Design review of the part built by this model. Coordinates are the model's own, in mm. Face numbers are marked on the shaded views. A direction names the side the tool comes from. Give positions to 0.01 mm unless a question says otherwise; leave off trailing zeros. Write each loop counter-clockwise with the first axis right and the second up, starting at its lowest first coordinate (ties: lowest second). Pieces come first, ordered by that corner, then holes. Notation, with made-up numbers: (-22.75, 59.25) -> (31.25, 59.25) arc R18 cw to (31.25, 80.25) -> close; hole circle Ø3 at (-11.75, -20.5). An arc over 180 degrees is marked (long way). Write each question's results on one line, items separated by ' | '. Start each with the question number.
(1) For the marked faces 4 and 5, list the 3-axis set-ups (+Z, -Z, +X, -X, +Y, -Y) from which the entire face can be reached by the end or side of a thin tool; tool diameter is ignored.
(2) To check wall thickness, follow probe 1 along X at (y, z) = (3, 18.25); probe 2 along Y at (x, z) = (13, 17); probe 3 along Z at (x, y) = (-26.5, -6). State the ranges of each line that lie inside material, in increasing order.
(3) Take a section at B-B (x = 3). Count the separate pieces of the cut face and the enclosed holes in it, plus the area to 3 significant figures.
(4) Take a section at C-C (y = 8.5). State the section outline as (x, z) points, plus the area to 3 significant figures.
(5) Take a section at A-A (z = 17.75). State the section outline as (x, y) points, plus the area to 3 significant figures.
(6) Mouldability with a two-part tool opening along Y and no side actions: class the marked faces 1, 2 and 3 as released by +Y, released by -Y, zero draft, split by the parting line, or undercut.
(7) Clearance check with flat-ended pins moving along their axes: pin 1 (6 mm diameter, centred on y = 3.5, z = 11.5, fed in from -X); pin 2 (1.2 mm diameter, centred on x = 30.5, y = -8.5, fed in from -Z). State where each tip first meets the part, or that it passes through.
from build123d import *

# Parameters (mm, degrees)
SKETCH1_W           = 61.7
SKETCH1_H           = 31.7
SKETCH1_W_2         = 58.7
SKETCH1_H_2         = 28.7
BOSS_EXTRUDE1_DEPTH = 19
SKETCH2_W           = 61.7
SKETCH2_H           = 31.7
BOSS_EXTRUDE2_DEPTH = 1
BOSS_EXTRUDE3_DEPTH = 5
CUT_EXTRUDE4_DEPTH  = 2
CUT_EXTRUDE2_DEPTH  = 32.7
CUT_EXTRUDE3_DEPTH  = 62.7
SKETCH9_W           = 7
SKETCH9_H           = 8.75
CUT_EXTRUDE5_DEPTH  = 62.7


with BuildPart() as part:
    # Sketch1 → Boss-Extrude1 (new body)
    with BuildSketch(Plane.XY):
        Rectangle(SKETCH1_W, SKETCH1_H)
        Rectangle(SKETCH1_W_2, SKETCH1_H_2, mode=Mode.SUBTRACT)
    extrude(amount=BOSS_EXTRUDE1_DEPTH)

    # Sketch2 → Boss-Extrude2 (add)
    with BuildSketch(Plane.XY.offset(19)):
        Rectangle(SKETCH2_W, SKETCH2_H)
    extrude(amount=BOSS_EXTRUDE2_DEPTH)

    # Sketch3 → Boss-Extrude3 (add)
    with BuildSketch(Plane(origin=(0, 0, 0), x_dir=(-1, 0, 0), z_dir=(0, 0, -1))):
        Polygon((-30.85, -15.85), (30.85, -15.85), (30.85, 15.85), (9, 15.85), (9, 14.35), (29.35, 14.35), (29.35, -14.35), (-29.35, -14.35), (-29.35, 14.35), (-9, 14.35), (-9, 15.85), (-30.85, 15.85), align=None)
    extrude(amount=BOSS_EXTRUDE3_DEPTH)

    # Sketch8 → Cut-Extrude4 (cut, through all)
    with BuildSketch(Plane(origin=(0, 0, 19), x_dir=(-1, 0, 0), z_dir=(0, 0, -1))):
        with BuildLine():
            Line((12, 6.5), (22, 6.5))
            ThreePointArc((22, 6.5), (24, 8.5), (22, 10.5))
            Line((22, 10.5), (12, 10.5))
            ThreePointArc((12, 10.5), (10, 8.5), (12, 6.5))
        make_face()
        with BuildLine():
            Line((12, -2), (22, -2))
            ThreePointArc((22, -2), (24, 0), (22, 2))
            Line((22, 2), (12, 2))
            ThreePointArc((12, 2), (10, 0), (12, -2))
        make_face()
        with BuildLine():
            Line((12, -10.5), (22, -10.5))
            ThreePointArc((22, -10.5), (24, -8.5), (22, -6.5))
            Line((22, -6.5), (12, -6.5))
            ThreePointArc((12, -6.5), (10, -8.5), (12, -10.5))
        make_face()
        with BuildLine():
            Line((-5, -10.5), (5, -10.5))
            ThreePointArc((5, -10.5), (7, -8.5), (5, -6.5))
            Line((5, -6.5), (-5, -6.5))
            ThreePointArc((-5, -6.5), (-7, -8.5), (-5, -10.5))
        make_face()
        with BuildLine():
            Line((-22, -10.5), (-12, -10.5))
            ThreePointArc((-12, -10.5), (-10, -8.5), (-12, -6.5))
            Line((-12, -6.5), (-22, -6.5))
            ThreePointArc((-22, -6.5), (-24, -8.5), (-22, -10.5))
        make_face()
        with BuildLine():
            Line((-22, -2), (-12, -2))
            ThreePointArc((-12, -2), (-10, 0), (-12, 2))
            Line((-12, 2), (-22, 2))
            ThreePointArc((-22, 2), (-24, 0), (-22, -2))
        make_face()
        with BuildLine():
            Line((-5, 6.5), (5, 6.5))
            ThreePointArc((5, 6.5), (7, 8.5), (5, 10.5))
            Line((5, 10.5), (-5, 10.5))
            ThreePointArc((-5, 10.5), (-7, 8.5), (-5, 6.5))
        make_face()
        with BuildLine():
            Line((-22, 6.5), (-12, 6.5))
            ThreePointArc((-12, 6.5), (-10, 8.5), (-12, 10.5))
            Line((-12, 10.5), (-22, 10.5))
            ThreePointArc((-22, 10.5), (-24, 8.5), (-22, 6.5))
        make_face()
        with BuildLine():
            Line((-5, -2), (5, -2))
            ThreePointArc((5, -2), (7, 0), (5, 2))
            Line((5, 2), (-5, 2))
            ThreePointArc((-5, 2), (-7, 0), (-5, -2))
        make_face()
    extrude(amount=-CUT_EXTRUDE4_DEPTH, mode=Mode.SUBTRACT)

    # Sketch5 → Cut-Extrude2 (cut, through all)
    with BuildSketch(Plane(origin=(-15, 15.85, 0), x_dir=(1, 0, 0), z_dir=(0, -1, 0))):
        with BuildLine():
            Line((-9.5, 4), (0.5, 4))
            ThreePointArc((0.5, 4), (2.5, 2), (0.5, 0))
            Line((0.5, 0), (-9.5, 0))
            ThreePointArc((-9.5, 0), (-11.5, 2), (-9.5, 4))
        make_face()
        with BuildLine():
            Line((10, 0), (20, 0))
            ThreePointArc((20, 0), (22, 2), (20, 4))
            Line((20, 4), (10, 4))
            ThreePointArc((10, 4), (8, 2), (10, 0))
        make_face()
        with BuildLine():
            Line((29.5, 0), (39.5, 0))
            ThreePointArc((39.5, 0), (41.5, 2), (39.5, 4))
            Line((39.5, 4), (29.5, 4))
            ThreePointArc((29.5, 4), (27.5, 2), (29.5, 0))
        make_face()
        with BuildLine():
            Line((10, 11), (20, 11))
            ThreePointArc((20, 11), (22, 13), (20, 15))
            Line((20, 15), (10, 15))
            ThreePointArc((10, 15), (8, 13), (10, 11))
        make_face()
        with BuildLine():
            Line((29.5, 11), (39.5, 11))
            ThreePointArc((39.5, 11), (41.5, 13), (39.5, 15))
            Line((39.5, 15), (29.5, 15))
            ThreePointArc((29.5, 15), (27.5, 13), (29.5, 11))
        make_face()
        with BuildLine():
            Line((-9.5, 11), (0.5, 11))
            ThreePointArc((0.5, 11), (2.5, 13), (0.5, 15))
            Line((0.5, 15), (-9.5, 15))
            ThreePointArc((-9.5, 15), (-11.5, 13), (-9.5, 11))
        make_face()
    extrude(amount=CUT_EXTRUDE2_DEPTH, mode=Mode.SUBTRACT)

    # Sketch7 → Cut-Extrude3 (cut, through all)
    with BuildSketch(Plane(origin=(30.85, -15, 0), x_dir=(0, 0, -1), z_dir=(-1, 0, 0))):
        with BuildLine():
            Line((-15, -26.5), (-15, -19.5))
            ThreePointArc((-15, -19.5), (-13, -17.5), (-11, -19.5))
            Line((-11, -19.5), (-11, -26.5))
            ThreePointArc((-11, -26.5), (-13, -28.5), (-15, -26.5))
        make_face()
        with BuildLine():
            Line((0, -26.5), (0, -19.5))
            ThreePointArc((0, -19.5), (-2, -17.5), (-4, -19.5))
            Line((-4, -19.5), (-4, -26.5))
            ThreePointArc((-4, -26.5), (-2, -28.5), (0, -26.5))
        make_face()
        with BuildLine():
            Line((0, -10.5), (0, -3.5))
            ThreePointArc((0, -3.5), (-2, -1.5), (-4, -3.5))
            Line((-4, -3.5), (-4, -10.5))
            ThreePointArc((-4, -10.5), (-2, -12.5), (0, -10.5))
        make_face()
        with BuildLine():
            Line((-11, -10.5), (-11, -3.5))
            ThreePointArc((-11, -3.5), (-13, -1.5), (-15, -3.5))
            Line((-15, -3.5), (-15, -10.5))
            ThreePointArc((-15, -10.5), (-13, -12.5), (-11, -10.5))
        make_face()
    extrude(amount=CUT_EXTRUDE3_DEPTH, mode=Mode.SUBTRACT)

    # Sketch9 → Cut-Extrude5 (cut, through all)
    with BuildSketch(Plane.ZY.offset(30.85)):
        with Locations((-1.5, 7.875)):
            Rectangle(SKETCH9_W, SKETCH9_H)
        with Locations((-1.5, -7.875)):
            Rectangle(SKETCH9_W, SKETCH9_H)
    extrude(amount=-CUT_EXTRUDE5_DEPTH, mode=Mode.SUBTRACT)


solid = part.part
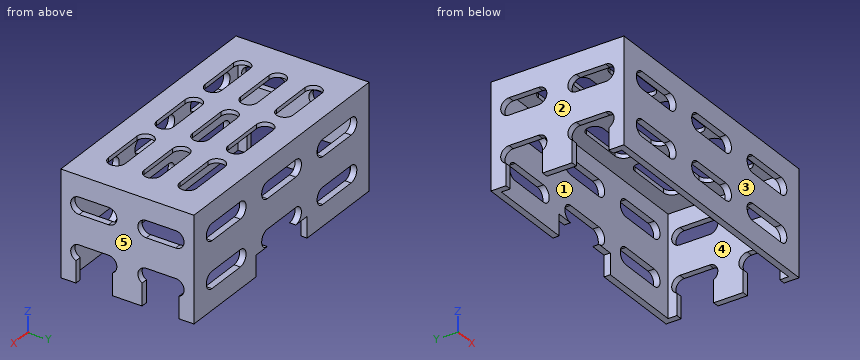
Report:
1) face 4: -Z | face 5: +Z, -Z, +X, +Y, -Y
2) probe 1: -30.85 to -29.35, 29.35 to 30.85 | probe 2: -15.85 to -14.35, 14.35 to 15.85 | probe 3: 19 to 20
3) separate pieces: 7 | enclosed holes: 0 | area: 60.2 mm2
4) outline: (-30.85, 4) -> (-29.35, 4) -> (-29.35, 11) -> (-30.85, 11) -> close; (-30.85, 15) -> (-29.35, 15) -> (-29.35, 19) -> (-24, 19) -> (-24, 20) -> (-30.85, 20) -> close; (-10, 19) -> (-7, 19) -> (-7, 20) -> (-10, 20) -> close; (7, 19) -> (10, 19) -> (10, 20) -> (7, 20) -> close; (24, 19) -> (29.35, 19) -> (29.35, 15) -> (30.85, 15) -> (30.85, 20) -> (24, 20) -> close; (29.35, 4) -> (30.85, 4) -> (30.85, 11) -> (29.35, 11) -> close | area: 52.7 mm2
5) outline: (-30.85, -15.85) -> (30.85, -15.85) -> (30.85, 15.85) -> (-30.85, 15.85) -> close; hole (-29.35, -14.35) -> (29.35, -14.35) -> (29.35, 14.35) -> (-29.35, 14.35) -> close | area: 271 mm2
6) face 1: undercut | face 2: zero draft | face 3: released by -Y
7) pin 1: x = -30.85 | pin 2: z = 4
